Can you work these out from the model? Positions are in its coordinate system, mm. Face numbers are marked on the shaded views. A direction names the side the tool comes from. Give positions to 0.01 mm unless a question says otherwise; leave off trailing zeros. Order: outer loops, then holes, each group sorted by start corner. A loop starts at its lowest first (then second) coordinate and runs counter-clockwise, first axis right, second up.
```python
from build123d import *

# Parameters (mm, degrees)
SKETCH1_W           = 138.1125
SKETCH1_H           = 39.6875
SKETCH1_W_2         = 131.7625
SKETCH1_H_2         = 33.3375
BOSS_EXTRUDE1_DEPTH = 14.2875
SKETCH2_W           = 138.1125
SKETCH2_H           = 39.6875
BOSS_EXTRUDE2_DEPTH = 3.175
CUT_EXTRUDE1_REACH  = 142.26
SKETCH3_W           = 14.2875
SKETCH3_H           = 33.3375
BOSS_EXTRUDE3_REACH = 142.26
SKETCH4_W           = 2.38125
SKETCH4_H           = 2.38125
BOSS_EXTRUDE4_START = -8.73125
SKETCH6_W           = 138.1125
SKETCH6_H           = 12.7
SKETCH6_R           = 2.5
BOSS_EXTRUDE4_DEPTH = 1.5
SKETCH7_R           = 2.95
CUT_EXTRUDE2_DEPTH  = 1
SKETCH8_R           = 63.5
BOSS_EXTRUDE5_DEPTH = 3.175
FILLET1_R           = 12.7
BOSS_EXTRUDE6_DEPTH = 36.5125


with BuildPart() as part:
    # Sketch1 → Boss-Extrude1 (new body)
    with BuildSketch(Plane.XY):
        Rectangle(SKETCH1_W, SKETCH1_H)
        Rectangle(SKETCH1_W_2, SKETCH1_H_2, mode=Mode.SUBTRACT)
    extrude(amount=BOSS_EXTRUDE1_DEPTH)

    # Sketch2 → Boss-Extrude2 (add)
    with BuildSketch(Plane(origin=(0, 0, 0), x_dir=(-1, 0, 0), z_dir=(0, 0, -1))):
        Rectangle(SKETCH2_W, SKETCH2_H)
    extrude(amount=BOSS_EXTRUDE2_DEPTH)

    # Sketch3 → Cut-Extrude1 (cut, up to next)
    with BuildSketch(Plane(origin=(69.05625, 0, 0), x_dir=(0, 0, -1), z_dir=(1, 0, 0)), mode=Mode.PRIVATE) as cut_extrude1_sk1:
        with Locations((-7.14375, 0)):
            Rectangle(SKETCH3_W, SKETCH3_H)
    cut_extrude1_tool1 = extrude(cut_extrude1_sk1.sketch, amount=-CUT_EXTRUDE1_REACH, mode=Mode.PRIVATE) & part.part
    add(cut_extrude1_tool1.solids().sort_by_distance((69.05625, 0, 7.14375))[0], mode=Mode.SUBTRACT)

    # Sketch4 → Boss-Extrude3 (add, up to next)
    with BuildSketch(Plane(origin=(69.05625, 0, 0), x_dir=(0, 0, -1), z_dir=(1, 0, 0)), mode=Mode.PRIVATE) as boss_extrude3_sk1:
        with Locations((-5.953125, -15.478125)):
            Rectangle(SKETCH4_W, SKETCH4_H)
    boss_extrude3_tool1 = extrude(boss_extrude3_sk1.sketch, amount=-BOSS_EXTRUDE3_REACH, mode=Mode.PRIVATE) - part.part
    # Sketch4 → Boss-Extrude3 (add, up to next)
    with BuildSketch(Plane(origin=(69.05625, 0, 0), x_dir=(0, 0, -1), z_dir=(1, 0, 0)), mode=Mode.PRIVATE) as boss_extrude3_sk2:
        with Locations((-5.953125, 15.478125)):
            Rectangle(SKETCH4_W, SKETCH4_H)
    boss_extrude3_tool2 = extrude(boss_extrude3_sk2.sketch, amount=-BOSS_EXTRUDE3_REACH, mode=Mode.PRIVATE) - part.part
    add(boss_extrude3_tool1.solids().sort_by_distance((69.05625, -15.478125, 5.953125))[0])
    add(boss_extrude3_tool2.solids().sort_by_distance((69.05625, 15.478125, 5.953125))[0])

    # Sketch6 → Boss-Extrude4 (add, symmetric)
    with BuildSketch(Plane(origin=(0, 0, -3.175), x_dir=(-1, 0, 0), z_dir=(0, 0, -1)).offset(BOSS_EXTRUDE4_START)):
        with Locations((0, 26.19375)):
            Rectangle(SKETCH6_W, SKETCH6_H)
        with Locations((0, 26.19375)):
            Circle(SKETCH6_R, mode=Mode.SUBTRACT)
        with Locations((-34.528125, 26.19375)):
            Circle(SKETCH6_R, mode=Mode.SUBTRACT)
        with Locations((34.528125, 26.19375)):
            Circle(SKETCH6_R, mode=Mode.SUBTRACT)
    extrude(amount=BOSS_EXTRUDE4_DEPTH, both=True)

    # Sketch7 → Cut-Extrude2 (cut)
    with BuildSketch(Plane(origin=(0, 0, 4.05625), x_dir=(-1, 0, 0), z_dir=(0, 0, -1))):
        with Locations((-34.528125, 26.19375)):
            Circle(SKETCH7_R)
        with Locations((0, 26.19375)):
            Circle(SKETCH7_R)
        with Locations((34.528125, 26.19375)):
            Circle(SKETCH7_R)
    extrude(amount=-CUT_EXTRUDE2_DEPTH, mode=Mode.SUBTRACT)

    # Sketch8 → Boss-Extrude5 (add)
    with BuildSketch(Plane.XZ.offset(19.84375)):
        with Locations((0, -49.2125)):
            Circle(SKETCH8_R)
    extrude(amount=-BOSS_EXTRUDE5_DEPTH)

    # Fillet1
    fillet1_edges = [part.edges().sort_by_distance(p)[0] for p in [
        (-43.735552972, -18.25625, -3.175),
        (43.735552972, -18.25625, -3.175),
    ]]
    fillet(fillet1_edges, radius=FILLET1_R)

    # Sketch10 → Boss-Extrude6 (add)
    with BuildSketch(Plane(origin=(0, -16.66875, 0), x_dir=(1, 0, 0), z_dir=(0, 1, 0))):
        with BuildLine():
            Line((-68.520442889, 3.175), (-58.995442889, 3.175))
            ThreePointArc((-58.995442889, 3.175), (-53.090093775, 12.144054919), (-54.245350621, 22.8203125))
            ThreePointArc((-54.245350621, 22.8203125), (0, 109.5375), (54.245350621, 22.8203125))
            ThreePointArc((54.245350621, 22.8203125), (53.090093775, 12.144054919), (58.995442889, 3.175))
            Line((58.995442889, 3.175), (68.520442889, 3.175))
            ThreePointArc((68.520442889, 3.175), (57.753494041, 9.139807909), (57.100369074, 21.43125))
            ThreePointArc((57.100369074, 21.43125), (0, 112.7125), (-57.100369074, 21.43125))
            ThreePointArc((-57.100369074, 21.43125), (-57.753494041, 9.139807909), (-68.520442889, 3.175))
        make_face()
    extrude(amount=BOSS_EXTRUDE6_DEPTH)


solid = part.part
```
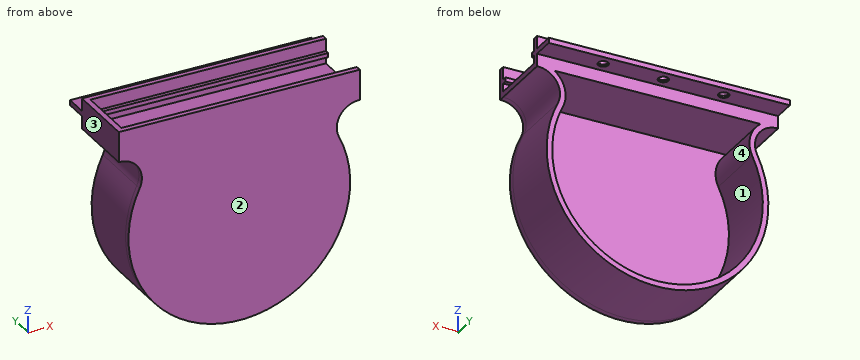
1) We'd pull the mould along Z, two halves only. Please class the marked faces 3 and 4: +Z half, -Z half, draft (parallel to the pull), parting line (faces both ways), or undercut.
2) Suppose I cut it at C-C (x = 15). Please give me the cut outline in (y, z) (1 decimal).
3) Suppose I cut it at D-D (z = -37). Please give me the cut outline in (x, y).
4) Which directions (+Z, -Z, +X, -X, +Y, -Y) give clear straight access to the entire face, cutting with the end or side of a thin tool? Please do the marked faces 1 and 2.
5) I'm going to push flat-ended pins straight in: pin 1 Ø4.5 at (x, y) = (-0.5, 25.5) entering from -Z; pin 2 Ø8 at (y, z) = (8, -97) entering from +X; pin 3 Ø6.5 at (x, y) = (0, 26.19) entering from +Z. Where does each tip first touch, or does it pass through?
6) If I drill on line 1 (X direction, y = -11.5, z = -15); line 2 (Y direction, x = -45, z = 3.5); line 3 (Y direction, x = 63.5, z = -1), over which ranges is the centre line in solid material (lowest first)?
Results:
1. face 3: draft
1. face 4: undercut
2. outline: (-19.8, -110.9) - (19.8, -110.9) - (19.8, -107.6) - (-16.7, -107.6) - (-16.7, -3.2) - (19.8, -3.2) - (19.8, 4.1) - (32.5, 4.1) - (32.5, 7.1) - (19.8, 7.1) - (19.8, 14.3) - (16.7, 14.3) - (16.7, 7.1) - (14.3, 7.1) - (14.3, 4.8) - (16.7, 4.8) - (16.7, 0) - (-16.7, 0) - (-16.7, 4.8) - (-14.3, 4.8) - (-14.3, 7.1) - (-16.7, 7.1) - (-16.7, 14.3) - (-19.8, 14.3) - close
3. outline: (-62.31, -19.84) - (62.31, -19.84) - (62.31, 19.84) - (59.08, 19.84) - (59.08, -16.67) - (-59.08, -16.67) - (-59.08, 19.84) - (-62.31, 19.84) - close
4. face 1: +Y
4. face 2: +Z, -Z, +X, -X, -Y
5. pin 1: stops at z = 4.06
5. pin 2: stops at x = 45.99
5. pin 3: stops at z = 7.06
6. line 1: x = -55.85 to -52.67, 52.67 to 55.85
6. line 2: y = -19.84 to -16.67, 16.67 to 19.84
6. line 3: y = -19.84 to 19.84
